Design review of the part built by this model. Coordinates are the model's own, in mm. A direction names the side the tool comes from. Give positions to 0.01 mm unless a question says otherwise; leave off trailing zeros. Loops run counter-clockwise (first coordinate to the right, second up) from the corner with the lowest first, then second, coordinate; pieces in that order, holes last. Notation, with made-up numbers: M 6,71 L 26,71 A31 ccw 26,104 Z; hole C 19.5,34.25 d6. An arc over 180 degrees is marked long. Use CSV: the item, a comma, the result in double quotes.
from build123d import *

# Parameters (mm, degrees)
F3_DEPTH = 10
F5_DEPTH = 3
F7_DEPTH = 19


with BuildPart() as f1:
    # F0 (on Top) → F1 (revolve)
    with BuildSketch(Plane.XY):
        with BuildLine():
            Line((0, 0), (0, 50))
            ThreePointArc((0, 50), (-35.355339, 35.355339), (-50, 0))
            Line((-50, 0), (0, 0))
        make_face()
    revolve(axis=Axis((0, 25, 0), (0, -1, 0)))

    # F2 (on Front) → F3 (cut)
    with BuildSketch(Plane.XZ):
        Polygon((27.5, 22), (-27.5, 22), (-27.5, 4), (-27.5, -4), (-27.5, -22), (27.5, -22), (27.5, -4), (27.5, 4), align=None)
    extrude(amount=-F3_DEPTH, mode=Mode.SUBTRACT)

    # F4 (on Front) → F5 (cut)
    with BuildSketch(Plane.XZ):
        with BuildLine():
            Line((12.5, -25), (0, -25))
            Line((0, -25), (-12.5, -25))
            ThreePointArc((-12.5, -25), (0, -37.5), (12.5, -25))
        make_face()
        with BuildLine():
            Line((-12.5, 25), (0, 25))
            Line((0, 25), (12.5, 25))
            ThreePointArc((12.5, 25), (0, 37.5), (-12.5, 25))
        make_face()
    extrude(amount=-F5_DEPTH, mode=Mode.SUBTRACT)

    # F6 (on Front) → F7 (join)
    with BuildSketch(Plane.XZ):
        with BuildLine():
            Line((-27.5, 0), (-27.5, 4))
            ThreePointArc((-27.5, 4), (-31.5, 0), (-27.5, -4))
            Line((-27.5, -4), (-27.5, 0))
        make_face()
        with BuildLine():
            ThreePointArc((31.5, 0), (30.328427, 2.828427), (27.5, 4))
            Line((27.5, 4), (27.5, 0))
            Line((27.5, 0), (27.5, -4))
            ThreePointArc((27.5, -4), (30.328427, -2.828427), (31.5, 0))
        make_face()
    extrude(amount=F7_DEPTH)


solid = f1.part
(1) Clearance check with flat-ended pins moving along their axes: P1, Ø6, axis at x = -22, z = 18.5, coming from the -Y side; P2, Ø6, axis at y = -6.5, z = -1, coming from the +X side; P3, Ø14, axis at x = 1, z = 33, coming from the -Y side. State where each tip first meets the part, or that it passes through.
A:
P1,"y = 10"
P2,"x = 31.5"
P3,"y = 0"
(2) Machinability: for faces 4 (the flat face through (-29, -19, 0)), 5 (the cylindrical face through (0.275, 1.479, 37.497)), which of the approach directions +Z, -Z, +X, -X, +Y, -Y give a long, thin tool a straight path to every point of the face, cutting with its end or side? Answer none if there is none.
A:
face 4,"+Z, -Z, +X, -X, -Y"
face 5,"-Y"
(3) Wall thickness on line 1 along Z through (x, y) = (-15, 4.5); line 2 along Z through (x, y) = (11.5, 4.5); line 3 along Y through (x, z) = (-10, -22.5): over which ranges is each line inside the solid? List them lowest first. Write a range as [from, to].
A:
line 1,"[-47.48, -22], [22, 47.48]"
line 2,"[-48.45, -22], [22, 48.45]"
line 3,"[0, 43.52]"
(4) The part is to be moulded in two halves that separate along Z. For faces 1 (the flat face through (1, 0, -23)), 2 (the flat face through (0, 5, -22)), 3 (the cylindrical face through (-31.5, -9.4, 0.1)), say which applies: released by +Z, released by -Z, zero draft, split by the parting line, or undercut.
A:
face 1,"zero draft"
face 2,"undercut"
face 3,"split by the parting line"
(5) We need section A-A on y = -10. State the section outline as (x, z) points, then the cut area to 3 significant figures.
A:
outline,"M -27.5,-4 L -27.5,4 A4 ccw Z; M 27.5,-4 A4 ccw 27.5,4 Z"
area,"50.3 mm²"
